```python
from build123d import *

# Parameters (mm, degrees)
CROQUIS1_W                        = 12.5
CROQUIS1_H                        = 13
CORTAR_EXTRUIR1_START             = -0.2
CORTAR_EXTRUIR1_DEPTH             = 0.2
DI_METRO_DE_TALADRO_5_0_5_1_D     = 5
DI_METRO_DE_TALADRO_5_0_5_1_DEPTH = 9
CHAFL_N1_SIZE                     = 0.2
CROQUIS5_R                        = 2.5
SALIENTE_EXTRUIR1_DEPTH           = 10


with BuildPart() as part:
    # Croquis1 → Revolución1 (revolve)
    with BuildSketch(Plane(origin=(0, 0, 0), x_dir=(-1, 0, 0), z_dir=(0, 0, -1)), mode=Mode.PRIVATE) as revoluci_n1_sk:
        with Locations((-6.25, 6.5)):
            Rectangle(CROQUIS1_W, CROQUIS1_H)
    revolve(revoluci_n1_sk.sketch.rotate(Axis((0, 0, 0), (0, 1, 0)), 180), axis=Axis((0, 0, 0), (0, 1, 0)))

    # Croquis2 → Cortar-Extruir1 (cut)
    with BuildSketch(Plane(origin=(0, 13, 0), x_dir=(-1, 0, 0), z_dir=(0, 1, 0)).offset(CORTAR_EXTRUIR1_START)):
        with BuildLine():
            Line((0.25, -12.49749975), (0.25, -7))
            Line((0.25, -7), (-0.25, -7))
            Line((-0.25, -7), (-0.25, -12.49749975))
            ThreePointArc((-0.25, -12.49749975), (0, -12.5), (0.25, -12.49749975))
        make_face()
    extrude(amount=CORTAR_EXTRUIR1_DEPTH, mode=Mode.SUBTRACT)

    # Diámetro de taladro Ø5.0 (5)1
    with Locations(Plane(origin=(0, 0, 0), x_dir=(-1, 0, 0), z_dir=(0, -1, 0))):
        with Locations((0, 0)):
            Hole(DI_METRO_DE_TALADRO_5_0_5_1_D / 2, depth=DI_METRO_DE_TALADRO_5_0_5_1_DEPTH)

    # Chaflán1
    chafl_n1_edges = [part.edges().sort_by_distance(p)[0] for p in [
        (8.75, 13, 8.926785536),
    ]]
    chamfer(chafl_n1_edges, length=CHAFL_N1_SIZE)

    # Croquis5 → Saliente-Extruir1 (add)
    with BuildSketch(Plane(origin=(0, 13, 0), x_dir=(-1, 0, 0), z_dir=(0, 1, 0))):
        with BuildLine():
            Line((0.25, -7), (-0.25, -7))
            Line((-0.25, -7), (-0.25, -12.49749975))
            ThreePointArc((-0.25, -12.49749975), (0, 12.5), (0.25, -12.49749975))
            Line((0.25, -12.49749975), (0.25, -7))
        make_face()
        with Locations(Location((0, 0, 0), (0, 0, 270))):
            Circle(CROQUIS5_R, mode=Mode.SUBTRACT)
    extrude(amount=-SALIENTE_EXTRUIR1_DEPTH)

    # Chaflán2: read off the stored shape, not the designer's step
    # Chaflán2 outline → Chaflán2 (revolve, cut)
    with BuildSketch(Plane.XY):
        Polygon((12.5, 13), (12, 13), (12.5, 12.5), align=None)
    revolve(axis=Axis((0, 0, 0), (0, 1, 0)), mode=Mode.SUBTRACT)


solid = part.part
```
For this review, take the finished solid that the model builds, in its own axes (mm). A direction names the side the tool comes from. Round coordinates to 2 decimals unless told otherwise and drop trailing zeros. Order: outer loops, then holes, each group sorted by start corner. A loop starts at its lowest first (then second) coordinate and runs counter-clockwise, first axis right, second up.
Q1. Wall thickness on line 1 (Z direction, x = 0, y = 5.5); line 2 (Z direction, x = 0.5, y = 3); line 3 (Z direction, x = 0, y = 10.5): over which ranges is each line inside the solid? List them lowest first.
Findings below:
line 1: z = -12.5 to -2.5, 2.5 to 12.5
line 2: z = -12.49 to -2.45, 2.45 to 12.49
line 3: z = -12.5 to 12.5
Q2. We need section C-C, the plane y = 10.75. Give the boundary of the cut face in (x, z), plus the area to 3 significant figures.
Findings below:
outline: circle Ø25 at (0, 0)
area: 491 mm2
Q3. Insertion check: P1, Ø2.5, axis at x = -0.5, z = 0.5, coming from the -Y side. The pin has a flat end and moves straight along its axis. Give the tip position at first contact, or say it passes through.
Findings below:
P1: stops at y = 9
Q4. Machinability: for faces 1 (the flat face through (0, 13, 0)), 2 (the cylindrical face through (-0.54, 4.56, 2.44)), which of the approach directions +Z, -Z, +X, -X, +Y, -Y give a long, thin tool a straight path to every point of the face, cutting with its end or side? Answer none if there is none.
Findings below:
face 1: +Z, -Z, +X, -X, +Y
face 2: -Y
Q5. We need section B-B, the plane y = 7.5. Give the boundary of the cut face in (x, z), plus the area to 3 significant figures.
Findings below:
outline: circle Ø25 at (0, 0); hole circle Ø5 at (0, 0)
area: 471 mm2
Q6. We need section A-A, the plane z = 0. Give the boundary of the cut face in (x, y).
Findings below:
outline: (-12.5, 0) - (-2.5, 0) - (-2.5, 9) - (2.5, 9) - (2.5, 0) - (12.5, 0) - (12.5, 12.5) - (12, 13) - (-12, 13) - (-12.5, 12.5) - close
Q7. Mouldability with a two-part tool opening along Z and no side actions: class faces 3 (the cylindrical face through (-11.923, 6.338, 3.755)), 4 (the flat face through (0, 9, 0)), 5 (the flat face through (0, 0, -3)) as pulls with the +Z half, pulls with the -Z half, needs draft (parallel to the pull), parting line crosses it, or undercut.
Findings below:
face 3: parting line crosses it
face 4: undercut
face 5: needs draft
